```python
from build123d import *

# Parameters (mm, degrees)
SKETCH1_W           = 50
SKETCH1_H           = 15
BOSS_EXTRUDE1_DEPTH = 3
FILLET2_R           = 2


with BuildPart() as part:
    # Sketch1 → Boss-Extrude1 (new body)
    with BuildSketch(Plane(origin=(0, 0, 0), x_dir=(1, 0, 0), z_dir=(0, 1, 0))):
        with Locations((25, 7.5)):
            Rectangle(SKETCH1_W, SKETCH1_H)
    extrude(amount=BOSS_EXTRUDE1_DEPTH)

    # Fillet2
    fillet2_edges = [part.edges().sort_by_distance(p)[0] for p in [
        (25, 3, -15),
    ]]
    fillet(fillet2_edges, radius=FILLET2_R)


solid = part.part
```
Can you work these out from the model? Positions are in its coordinate system, mm. Give positions to 0.01 mm unless a question says otherwise; leave off trailing zeros. Loops run counter-clockwise (first coordinate to the right, second up) from the corner with the lowest first, then second, coordinate; pieces in that order, holes last. Notation, with made-up numbers: M 2.5,39 L 59.5,39 A12 cw 59.5,51 Z; hole C 50.25,57 d6. An arc over 180 degrees is marked long. Answer in a Markdown table with one row per item.
1. Suppose I cut it at B-B on y = 2.15. Write out the boundary of the cut face in (x, z).
Taken from the geometry:
| item | result |
|---|---|
| outline | M 0,-14.64 L 50,-14.64 L 50,0 L 0,0 Z |
2. For pin 1 Ø1 at (y, z) = (1.5, -4) entering from -X, with a flat end and sliding along its axis, tell me the tip position at first contact or that it passes through.
Taken from the geometry:
| item | result |
|---|---|
| pin 1 | stops at x = 0 |
3. If I drill on line 1 along Y through (x, z) = (14.5, -13.5); line 2 along Z through (x, y) = (32.5, 1.4); line 3 along Z through (x, y) = (7, 2.1), over which ranges is the centre line in solid material (lowest first)?
Taken from the geometry:
| item | result |
|---|---|
| line 1 | y = 0 to 2.94 |
| line 2 | z = -14.96 to 0 |
| line 3 | z = -14.67 to 0 |
4. Suppose I cut it at A-A on x = 42. Write out the boundary of the cut face in (y, z), plus the area to 3 significant figures.
Taken from the geometry:
| item | result |
|---|---|
| outline | M 0,-15 L 1,-15 A2 ccw 3,-13 L 3,0 L 0,0 Z |
| area | 44.1 mm² |
